from build123d import *

# Parameters (mm, degrees)
F0_W           = 76.2
F0_H           = 50.8
F1_DEPTH       = 25.4
F2_R           = 12.7
F3_DEPTH       = 32.766
F5_DEPTH       = 25.4
F7_D           = 5.5
F7_DEPTH       = 254
F7_CBORE_D     = 9.75
F7_CBORE_DEPTH = 15
F7_TIP         = 1.6523667023
F8_DEPTH       = 2.54


with BuildPart() as f1:
    # F0 (on Front) → F1 (new body)
    with BuildSketch(Plane.XZ):
        Rectangle(F0_W, F0_H)
    extrude(amount=F1_DEPTH)

    # F2 (on face) → F3 (cut)
    with BuildSketch(Plane.XZ.offset(25.4)):
        Circle(F2_R)
    extrude(amount=-F3_DEPTH, mode=Mode.SUBTRACT)

    # F4 (on face) → F5 (cut)
    with BuildSketch(Plane.XZ.offset(25.4)):
        with BuildLine():
            ThreePointArc((1.5e-09, 25.4), (17.9605122427, 17.9605122416), (25.4, 0))
            Line((25.4, 0), (38.1, 0))
            Line((38.1, 0), (38.1, 25.4))
            Line((38.1, 25.4), (1.5e-09, 25.4))
        make_face()
        with BuildLine():
            ThreePointArc((-25.4, 0), (-17.9605122416, 17.9605122427), (1.5e-09, 25.4))
            Line((1.5e-09, 25.4), (-38.1, 25.4))
            Line((-38.1, 25.4), (-38.1, 0))
            Line((-38.1, 0), (-25.4, 0))
        make_face()
    extrude(amount=-F5_DEPTH, mode=Mode.SUBTRACT)

    # F7
    with Locations(Plane.XY):
        with Locations((-31.75, -6.35), (-31.75, -19.05), (31.75, -6.35), (31.75, -19.05)):
            CounterBoreHole(F7_D / 2, F7_CBORE_D / 2, F7_CBORE_DEPTH, depth=F7_DEPTH)
            with Locations((0, 0, -(F7_DEPTH + F7_TIP / 2))):  # 118° drill point
                Cone(0, F7_D / 2, F7_TIP, mode=Mode.SUBTRACT)

    # F8 (cut): a face of the model
    f8_faces = [f1.faces().sort_by_distance(p)[0] for p in [
        (0, -12.7, -25.4),
    ]]
    extrude(f8_faces, amount=-F8_DEPTH, mode=Mode.SUBTRACT)


solid = f1.part
Here's how the part is built. I have some questions about the finished solid (model axes, mm). A direction names the side the tool comes from. Give positions to 0.01 mm unless a question says otherwise; leave off trailing zeros. Loops run counter-clockwise (first coordinate to the right, second up) from the corner with the lowest first, then second, coordinate; pieces in that order, holes last. Notation, with made-up numbers: (-26.75, 20) -> (-2.75, 20) arc R23 ccw to (-2.75, 58) -> close; hole circle Ø4 at (58.25, 12). An arc over 180 degrees is marked (long way). Answer as a JSON object with one key per item and string values. Group by question number.
Item 1: I need wall thicknesses on L1, parallel to X at y = -19, z = -13.5; L2, parallel to Y at x = -31.75, z = -19.5; L3, parallel to Y at x = -31.75, z = -12 (3 decimals). Which ranges of each line are inside material? Lowest first, please.
Item 2: Imagine slicing it at D-D on y = -4.5. Write out the boundary of the cut face in (x, z).
Item 3: Will these pins go through, and if not, where does the flat tip stop? pin 1 (5 mm diameter, centred on x = 31.75, y = -19.05, fed in from -Z); pin 2 (6 mm diameter, centred on x = -31.75, y = -6.35, fed in from +Z); pin 3 (5 mm diameter, centred on y = -15, z = 8, fed in from -X); pin 4 (4 mm diameter, centred on x = -31, y = -16, fed in from +Z).
Item 4: Imagine slicing it at A-A on z = -1. Write out the boundary of the cut face in (x, y) (3 decimals).
Item 5: On a 3-axis mill with a long thin cutter (end or side, diameter ignored), from which of +Z, -Z, +X, -X, +Y, -Y can I reach the whole of each face in a straight line? I mean faces 5 (the flat face through (-32, -13, 0)), 6 (the flat face through (34, -21, -15)), 7 (the flat face through (32, -13, 0)). Say none if no direction works.
Item 6: Imagine slicing it at B-B on x = -31.75. Write out the boundary of the cut face in (y, z) (3 decimals).
Item 7: Imagine slicing it at C-C on y = -12.5. Write out the boundary of the cut face in (x, z), then the cut area to 3 significant figures.
Item 8: Thinking about a two-plate mould opening in Y: for faces 1 (the flat face through (-1, 0, -14)), 2 (the cylindrical face through (26.88, -18.84, -7.4)), 3 (the flat face through (-1, -13, -22.86)), 4 (the cylindrical face through (-36.62, -18.84, -7.4)), which applies, pulls with the +Y half, pulls with the -Y half, needs draft (parallel to the pull), parting line crosses it, or undercut?
Answer list:
{
 "1": {"L1": "x = -38.1 to -36.62, -26.88 to 26.88, 36.62 to 38.1", "L2": "y = -25.4 to -21.8, -16.3 to -9.1, -3.6 to 0", "L3": "y = -25.4 to -23.925, -14.175 to -11.225, -1.475 to 0"},
 "2": {"outline": "(-38.1, -22.86) -> (-33.78, -22.86) -> (-33.78, -15) -> (-36.26, -15) -> (-36.26, 0) -> (-38.1, 0) -> close; (-29.72, -22.86) -> (29.72, -22.86) -> (29.72, -15) -> (27.24, -15) -> (27.24, 0) -> (25.4, 0) arc R25.4 ccw to (-25.4, 0) -> (-27.24, 0) -> (-27.24, -15) -> (-29.72, -15) -> close; (33.78, -22.86) -> (38.1, -22.86) -> (38.1, 0) -> (36.26, 0) -> (36.26, -15) -> (33.78, -15) -> close; hole circle Ø25.4 at (0, 0)"},
 "3": {"pin 1": "passes through", "pin 2": "stops at z = -15", "pin 3": "stops at x = -24.8", "pin 4": "stops at z = 0"},
 "4": {"outline": "(-38.1, -25.4) -> (-12.661, -25.4) -> (-12.661, 0) -> (-38.1, 0) -> close; (12.661, -25.4) -> (38.1, -25.4) -> (38.1, 0) -> (12.661, 0) -> close; hole circle Ø9.75 at (-31.75, -19.05); hole circle Ø9.75 at (-31.75, -6.35); hole circle Ø9.75 at (31.75, -19.05); hole circle Ø9.75 at (31.75, -6.35)"},
 "5": {"face 5": "+Z, -X, +Y, -Y", "face 6": "+Z", "face 7": "+Z, +X, +Y, -Y"},
 "6": {"outline": "(-25.4, -22.86) -> (-21.8, -22.86) -> (-21.8, -15) -> (-23.925, -15) -> (-23.925, 0) -> (-25.4, 0) -> close; (-16.3, -22.86) -> (-9.1, -22.86) -> (-9.1, -15) -> (-11.225, -15) -> (-11.225, 0) -> (-14.175, 0) -> (-14.175, -15) -> (-16.3, -15) -> close; (-3.6, -22.86) -> (0, -22.86) -> (0, 0) -> (-1.475, 0) -> (-1.475, -15) -> (-3.6, -15) -> close"},
 "7": {"outline": "(-38.1, -22.86) -> (38.1, -22.86) -> (38.1, 0) -> (25.4, 0) arc R25.4 ccw to (-25.4, 0) -> (-38.1, 0) -> close; hole circle Ø25.4 at (0, 0)", "area": "2,250 mm2"},
 "8": {"face 1": "pulls with the +Y half", "face 2": "undercut", "face 3": "needs draft", "face 4": "undercut"}
}
